```python
from build123d import *

# Parameters (mm, degrees)
SKETCH_1_W          = 235
SKETCH_1_H          = 300
EXTRUDE_1_DEPTH     = 2
CUT_EXTRUDE_1_DEPTH = 191.552486208
SKETCH_5_W          = 20
SKETCH_5_H          = 80
SKETCH_5_H_2        = 40
CUT_EXTRUDE_2_DEPTH = 191.552486208
FILLET_1_R          = 3


with BuildPart() as part:
    # 草图1 → 凸台-拉伸1 (new body)
    with BuildSketch(Plane.XY):
        Rectangle(SKETCH_1_W, SKETCH_1_H)
    extrude(amount=EXTRUDE_1_DEPTH)

    # 草图4 → 切除-拉伸1 (cut, through all)
    with BuildSketch(Plane.XY.offset(2)):
        with BuildLine():
            Line((-103.3, 125), (-103.3, -125))
            ThreePointArc((-103.3, -125), (-107.5, -129.2), (-111.7, -125))
            Line((-111.7, -125), (-111.7, 125))
            ThreePointArc((-111.7, 125), (-107.5, 129.2), (-103.3, 125))
        make_face()
        with BuildLine():
            Line((111.7, 130), (111.7, 110))
            ThreePointArc((111.7, 110), (107.5, 105.8), (103.3, 110))
            Line((103.3, 110), (103.3, 130))
            ThreePointArc((103.3, 130), (107.5, 134.2), (111.7, 130))
        make_face()
        with BuildLine():
            Line((103.3, 90), (103.3, 70))
            ThreePointArc((103.3, 70), (107.5, 65.8), (111.7, 70))
            Line((111.7, 70), (111.7, 90))
            ThreePointArc((111.7, 90), (107.5, 94.2), (103.3, 90))
        make_face()
        with BuildLine():
            Line((103.3, 50), (103.3, 30))
            ThreePointArc((103.3, 30), (107.5, 25.8), (111.7, 30))
            Line((111.7, 30), (111.7, 50))
            ThreePointArc((111.7, 50), (107.5, 54.2), (103.3, 50))
        make_face()
        with BuildLine():
            Line((103.3, 10), (103.3, -10))
            ThreePointArc((103.3, -10), (107.5, -14.2), (111.7, -10))
            Line((111.7, -10), (111.7, 10))
            ThreePointArc((111.7, 10), (107.5, 14.2), (103.3, 10))
        make_face()
        with BuildLine():
            Line((103.3, -30), (103.3, -50))
            ThreePointArc((103.3, -50), (107.5, -54.2), (111.7, -50))
            Line((111.7, -50), (111.7, -30))
            ThreePointArc((111.7, -30), (107.5, -25.8), (103.3, -30))
        make_face()
        with BuildLine():
            Line((103.3, -70), (103.3, -90))
            ThreePointArc((103.3, -90), (107.5, -94.2), (111.7, -90))
            Line((111.7, -90), (111.7, -70))
            ThreePointArc((111.7, -70), (107.5, -65.8), (103.3, -70))
        make_face()
        with BuildLine():
            Line((103.3, -110), (103.3, -130))
            ThreePointArc((103.3, -130), (107.5, -134.2), (111.7, -130))
            Line((111.7, -130), (111.7, -110))
            ThreePointArc((111.7, -110), (107.5, -105.8), (103.3, -110))
        make_face()
        with BuildLine():
            Line((-80, 136), (-10, 136))
            ThreePointArc((-10, 136), (-4, 130), (-10, 124))
            Line((-10, 124), (-80, 124))
            ThreePointArc((-80, 124), (-86, 130), (-80, 136))
        make_face()
        with BuildLine():
            Line((-80, 104), (-10, 104))
            ThreePointArc((-10, 104), (-4, 110), (-10, 116))
            Line((-10, 116), (-80, 116))
            ThreePointArc((-80, 116), (-86, 110), (-80, 104))
        make_face()
        with BuildLine():
            Line((-80, 84), (-10, 84))
            ThreePointArc((-10, 84), (-4, 90), (-10, 96))
            Line((-10, 96), (-80, 96))
            ThreePointArc((-80, 96), (-86, 90), (-80, 84))
        make_face()
        with BuildLine():
            Line((-80, 64), (-10, 64))
            ThreePointArc((-10, 64), (-4, 70), (-10, 76))
            Line((-10, 76), (-80, 76))
            ThreePointArc((-80, 76), (-86, 70), (-80, 64))
        make_face()
        with BuildLine():
            Line((-80, 44), (-10, 44))
            ThreePointArc((-10, 44), (-4, 50), (-10, 56))
            Line((-10, 56), (-80, 56))
            ThreePointArc((-80, 56), (-86, 50), (-80, 44))
        make_face()
        with BuildLine():
            Line((-80, 24), (-10, 24))
            ThreePointArc((-10, 24), (-4, 30), (-10, 36))
            Line((-10, 36), (-80, 36))
            ThreePointArc((-80, 36), (-86, 30), (-80, 24))
        make_face()
        with BuildLine():
            Line((-80, 4), (-10, 4))
            ThreePointArc((-10, 4), (-4, 10), (-10, 16))
            Line((-10, 16), (-80, 16))
            ThreePointArc((-80, 16), (-86, 10), (-80, 4))
        make_face()
        with BuildLine():
            Line((-80, -16), (-10, -16))
            ThreePointArc((-10, -16), (-4, -10), (-10, -4))
            Line((-10, -4), (-80, -4))
            ThreePointArc((-80, -4), (-86, -10), (-80, -16))
        make_face()
        with BuildLine():
            Line((-80, -36), (-10, -36))
            ThreePointArc((-10, -36), (-4, -30), (-10, -24))
            Line((-10, -24), (-80, -24))
            ThreePointArc((-80, -24), (-86, -30), (-80, -36))
        make_face()
        with BuildLine():
            Line((-80, -56), (-10, -56))
            ThreePointArc((-10, -56), (-4, -50), (-10, -44))
            Line((-10, -44), (-80, -44))
            ThreePointArc((-80, -44), (-86, -50), (-80, -56))
        make_face()
        with BuildLine():
            Line((-80, -76), (-10, -76))
            ThreePointArc((-10, -76), (-4, -70), (-10, -64))
            Line((-10, -64), (-80, -64))
            ThreePointArc((-80, -64), (-86, -70), (-80, -76))
        make_face()
        with BuildLine():
            Line((-80, -96), (-10, -96))
            ThreePointArc((-10, -96), (-4, -90), (-10, -84))
            Line((-10, -84), (-80, -84))
            ThreePointArc((-80, -84), (-86, -90), (-80, -96))
        make_face()
        with BuildLine():
            Line((-80, -116), (-10, -116))
            ThreePointArc((-10, -116), (-4, -110), (-10, -104))
            Line((-10, -104), (-80, -104))
            ThreePointArc((-80, -104), (-86, -110), (-80, -116))
        make_face()
        with BuildLine():
            Line((-80, -136), (-10, -136))
            ThreePointArc((-10, -136), (-4, -130), (-10, -124))
            Line((-10, -124), (-80, -124))
            ThreePointArc((-80, -124), (-86, -130), (-80, -136))
        make_face()
        with BuildLine():
            Line((80, -124), (10, -124))
            ThreePointArc((10, -124), (4, -130), (10, -136))
            Line((10, -136), (80, -136))
            ThreePointArc((80, -136), (86, -130), (80, -124))
        make_face()
        with BuildLine():
            Line((80, -104), (10, -104))
            ThreePointArc((10, -104), (4, -110), (10, -116))
            Line((10, -116), (80, -116))
            ThreePointArc((80, -116), (86, -110), (80, -104))
        make_face()
        with BuildLine():
            Line((80, -84), (10, -84))
            ThreePointArc((10, -84), (4, -90), (10, -96))
            Line((10, -96), (80, -96))
            ThreePointArc((80, -96), (86, -90), (80, -84))
        make_face()
        with BuildLine():
            Line((80, -64), (10, -64))
            ThreePointArc((10, -64), (4, -70), (10, -76))
            Line((10, -76), (80, -76))
            ThreePointArc((80, -76), (86, -70), (80, -64))
        make_face()
        with BuildLine():
            Line((80, -44), (10, -44))
            ThreePointArc((10, -44), (4, -50), (10, -56))
            Line((10, -56), (80, -56))
            ThreePointArc((80, -56), (86, -50), (80, -44))
        make_face()
        with BuildLine():
            Line((80, -24), (10, -24))
            ThreePointArc((10, -24), (4, -30), (10, -36))
            Line((10, -36), (80, -36))
            ThreePointArc((80, -36), (86, -30), (80, -24))
        make_face()
        with BuildLine():
            Line((80, -4), (10, -4))
            ThreePointArc((10, -4), (4, -10), (10, -16))
            Line((10, -16), (80, -16))
            ThreePointArc((80, -16), (86, -10), (80, -4))
        make_face()
        with BuildLine():
            Line((80, 36), (10, 36))
            ThreePointArc((10, 36), (4, 30), (10, 24))
            Line((10, 24), (80, 24))
            ThreePointArc((80, 24), (86, 30), (80, 36))
        make_face()
        with BuildLine():
            Line((80, 16), (10, 16))
            ThreePointArc((10, 16), (4, 10), (10, 4))
            Line((10, 4), (80, 4))
            ThreePointArc((80, 4), (86, 10), (80, 16))
        make_face()
        with BuildLine():
            Line((80, 56), (10, 56))
            ThreePointArc((10, 56), (4, 50), (10, 44))
            Line((10, 44), (80, 44))
            ThreePointArc((80, 44), (86, 50), (80, 56))
        make_face()
        with BuildLine():
            Line((80, 76), (10, 76))
            ThreePointArc((10, 76), (4, 70), (10, 64))
            Line((10, 64), (80, 64))
            ThreePointArc((80, 64), (86, 70), (80, 76))
        make_face()
        with BuildLine():
            Line((80, 96), (10, 96))
            ThreePointArc((10, 96), (4, 90), (10, 84))
            Line((10, 84), (80, 84))
            ThreePointArc((80, 84), (86, 90), (80, 96))
        make_face()
        with BuildLine():
            Line((80, 116), (10, 116))
            ThreePointArc((10, 116), (4, 110), (10, 104))
            Line((10, 104), (80, 104))
            ThreePointArc((80, 104), (86, 110), (80, 116))
        make_face()
        with BuildLine():
            Line((80, 136), (10, 136))
            ThreePointArc((10, 136), (4, 130), (10, 124))
            Line((10, 124), (80, 124))
            ThreePointArc((80, 124), (86, 130), (80, 136))
        make_face()
    extrude(amount=-CUT_EXTRUDE_1_DEPTH, mode=Mode.SUBTRACT)

    # 草图5 → 切除-拉伸2 (cut, through all)
    with BuildSketch(Plane.XY.offset(2)):
        with Locations((107.5, -20)):
            Rectangle(SKETCH_5_W, SKETCH_5_H)
        with Locations((107.5, 80)):
            Rectangle(SKETCH_5_W, SKETCH_5_H_2)
    extrude(amount=-CUT_EXTRUDE_2_DEPTH, mode=Mode.SUBTRACT)

    # 圆角1
    fillet_1_edges = [part.edges().sort_by_distance(p)[0] for p in [
        (117.5, 20, 1),
        (117.5, -60, 1),
        (117.5, 100, 1),
        (117.5, 60, 1),
        (117.5, -150, 1),
        (-117.5, -150, 1),
        (-117.5, 150, 1),
        (117.5, 150, 1),
    ]]
    fillet(fillet_1_edges, radius=FILLET_1_R)


solid = part.part
```
The listing builds one solid part. Answer for the finished solid, in the listing's coordinates (mm). Give positions to 0.01 mm unless a question says otherwise; leave off trailing zeros. Order: outer loops, then holes, each group sorted by start corner. A loop starts at its lowest first (then second) coordinate and runs counter-clockwise, first axis right, second up. Notation, with made-up numbers: (61.25, -20) -> (117.25, -20) arc R26 cw to (117.25, -4) -> close; hole circle Ø11 at (39.5, 51.25). An arc over 180 degrees is marked (long way). Answer as CSV lines item,"result". Start each with the question number.
Q1. A cutting plane is placed at C-C (z = 0.5). Count the separate pieces of the cut face and the enclosed holes in it, then the cut area to 3 significant figures.
Q2. A cutting plane is placed at B-B (x = 107.5). Determine the outline of the cut face in (y, z).
Q3. A cutting plane is placed at A-A (y = -50). Determine the outline of the cut face in (x, z).
Q4. Find the intervals of material crossed by L1, parallel to X at y = 119, z = 1.95; L2, parallel to X at y = -38, z = 1.7; L3, parallel to X at y = -114.5, z = 1.85, in increasing order.
Q5. Determine the mould class of faces 1 (the cylindrical face through (-4, -70, 1)), 2 (the flat face through (-2, 2, 0)), 3 (the cylindrical face through (86, 30, 1)) for opening direction X: pulls with the +X half, pulls with the -X half, needs draft (parallel to the pull), parting line crosses it, or undercut.
Results found:
1,separate pieces,"1"
1,enclosed holes,"33"
1,area,"38,300 mm2"
2,outline,"(-150, 0) -> (-134.2, 0) -> (-134.2, 2) -> (-150, 2) -> close; (-105.8, 0) -> (-94.2, 0) -> (-94.2, 2) -> (-105.8, 2) -> close; (-65.8, 0) -> (-60, 0) -> (-60, 2) -> (-65.8, 2) -> close; (20, 0) -> (25.8, 0) -> (25.8, 2) -> (20, 2) -> close; (54.2, 0) -> (60, 0) -> (60, 2) -> (54.2, 2) -> close; (100, 0) -> (105.8, 0) -> (105.8, 2) -> (100, 2) -> close; (134.2, 0) -> (150, 0) -> (150, 2) -> (134.2, 2) -> close"
3,outline,"(-117.5, 0) -> (-111.7, 0) -> (-111.7, 2) -> (-117.5, 2) -> close; (-103.3, 0) -> (-86, 0) -> (-86, 2) -> (-103.3, 2) -> close; (-4, 0) -> (4, 0) -> (4, 2) -> (-4, 2) -> close; (86, 0) -> (97.5, 0) -> (97.5, 2) -> (86, 2) -> close"
4,L1,"-117.5 to -111.7, -103.3 to 103.3, 111.7 to 117.5"
4,L2,"-117.5 to -111.7, -103.3 to 97.5"
4,L3,"-117.5 to -111.7, -103.3 to -83.97, -6.03 to 6.03, 83.97 to 103.3, 111.7 to 117.5"
5,face 1,"undercut"
5,face 2,"needs draft"
5,face 3,"undercut"
